```python
from build123d import *

# Parameters (mm, degrees)
F1_DEPTH        = 10
F2_R            = 5
F3_R            = 3
F4_DEPTH        = 6
F4_COPIES_COUNT = 3


# Not quite as in the source:
# - a pattern or mirror of a feature is missing from the dataset's text; its kind, count and spacing are read off the source's solid


with BuildPart() as f1:
    # F0 (on Top) → F1 (new body)
    with BuildSketch(Plane.XY):
        Polygon((60, -34.6410161514), (0, 69.2820323028), (-60, -34.6410161514), align=None)
        Polygon((0, 57.735026919), (50, -28.8675134595), (-50, -28.8675134595), align=None, mode=Mode.SUBTRACT)
    extrude(amount=F1_DEPTH)

    # F2
    f2_edges = [f1.edges().sort_by_distance(p)[0] for p in [
        (-60, -34.641016, 5),
        (60, -34.641016, 5),
        (0, 69.282032, 5),
        (50, -28.867513, 5),
        (0, 57.735027, 5),
        (-50, -28.867513, 5),
    ]]
    fillet(f2_edges, radius=F2_R)

    # F3 (on face) → F4 (join)
    with BuildSketch(Plane.XZ.offset(34.6410161514)):
        with Locations((0, 5)):
            Circle(F3_R)
    f4 = extrude(amount=F4_DEPTH)

    # F4_copies: F4 ×3 about axis
    f4_copies_axis = Axis((0, 0, 0), (0, 0, 1))
    for i in range(1, F4_COPIES_COUNT):
        add(f4.rotate(f4_copies_axis, i * 360 / F4_COPIES_COUNT))


solid = f1.part
```
Design review of the part built by this model. Coordinates are the model's own, in mm. A direction names the side the tool comes from. Coordinates: 2 decimals unless noted, no trailing zeros. Order: outer loops, then holes, each group sorted by start corner. A loop starts at its lowest first (then second) coordinate and runs counter-clockwise, first axis right, second up. Notation, with made-up numbers: (8, 16.5) - (19, 16.5) arc R24 ccw to (19, 27.5) - close; hole circle Ø7 at (84, 75.25). An arc over 180 degrees is marked (long way). Answer in a Markdown table with one row per item.
(1) Consider section B-B on y = -1.5. State the section outline as (x, z) points.
Checked values:
| item | result |
|---|---|
| outline | (-40.87, 0) - (-34.2, 0) - (-34.2, 10) - (-40.87, 10) - close; (34.2, 0) - (40.87, 0) - (40.87, 10) - (34.2, 10) - close |
(2) Consider section D-D on x = -39. State the section outline as (y, z) points, plus the area to 3 significant figures.
Checked values:
| item | result |
|---|---|
| outline | (-34.64, 0) - (-28.87, 0) - (-28.87, 10) - (-34.64, 10) - close; (-9.81, 0) - (1.73, 0) - (1.73, 10) - (-9.81, 10) - close |
| area | 173 mm^2 |
(3) Clearance check with flat-ended pins moving along their axes: pin 1 (1 mm diameter, centred on x = 27.5, z = 5.5, fed in from -Y); pin 2 (3 mm diameter, centred on y = 18, z = 2, fed in from +X); pin 3 (5 mm diameter, centred on x = -15, z = 5, fed in from +Y). State where each tip first meets the part, or that it passes through.
Checked values:
| item | result |
|---|---|
| pin 1 | y = -34.64 |
| pin 2 | x = 36.49 |
| pin 3 | y = 47.63 |
(4) For faces 4 (the cylindrical face through (-45.71, -26.3, 5.07)), 5 (the cylindrical face through (-0.65, -37.6, 2.07)), 6 (the flat face through (-25, 15, 10)), list the 3-axis set-ups (+Z, -Z, +X, -X, +Y, -Y) from which the entire face can be reached by the end or side of a thin tool; tool diameter is ignored.
Checked values:
| item | result |
|---|---|
| face 4 | +Z, -Z |
| face 5 | -Y |
| face 6 | +Z, +X, -X, +Y, -Y |
(5) Consider section C-C on z = 5. State the section outline as (x, y) points.
Checked values:
| item | result |
|---|---|
| outline | (-55.67, -27.14) arc R5 ccw to (-51.34, -34.64) - (-3, -34.64) - (-3, -40.64) - (3, -40.64) - (3, -34.64) - (51.34, -34.64) arc R5 ccw to (55.67, -27.14) - (31.5, 14.72) - (36.7, 17.72) - (33.7, 22.92) - (28.5, 19.92) - (4.33, 61.78) arc R5 ccw to (-4.33, 61.78) - (-28.5, 19.92) - (-33.7, 22.92) - (-36.7, 17.72) - (-31.5, 14.72) - close; hole (-45.67, -21.37) arc R5 ccw to (-41.34, -28.87) - (41.34, -28.87) arc R5 ccw to (45.67, -21.37) - (4.33, 50.24) arc R5 ccw to (-4.33, 50.24) - close |
(6) Consider section A-A on x = 0. State the section outline as (y, z) points.
Checked values:
| item | result |
|---|---|
| outline | (-40.64, 2) - (-34.64, 2) - (-34.64, 0) - (-28.87, 0) - (-28.87, 10) - (-34.64, 10) - (-34.64, 8) - (-40.64, 8) - close; (52.74, 0) - (64.28, 0) - (64.28, 10) - (52.74, 10) - close |
(7) The part is to be moulded in two halves that separate along Y. For faces 1 (the flat face through (-1, -34.641, 2)), 2 (the flat face through (35.22, 20.28, 5.04)), 3 (the cylindrical face through (45.633, -26.431, 5.07)), say which applies: released by +Y, released by -Y, zero draft, split by the parting line, or undercut.
Checked values:
| item | result |
|---|---|
| face 1 | released by -Y |
| face 2 | released by +Y |
| face 3 | undercut |
(8) Wall thickness on line 1 along Y through (x, z) = (-32, 6.5); line 2 along X through (y, z) = (18, 6.75); line 3 along Y through (x, z) = (-15.5, 3.5): over which ranges is each line inside the solid? List them lowest first. Write a range as from..to.
Checked values:
| item | result |
|---|---|
| line 1 | -34.64..-28.87, 2.31..13.86, 15.48..21.48 |
| line 2 | -36.05..-22.94, 22.94..36.05 |
| line 3 | -34.64..-28.87, 30.89..42.44 |
